Could you check a few things on this drawing? It's one solid part, dimensions in mm from its lowest x, y, z. Give positions to 0.01 mm unless a question says otherwise; leave off trailing zeros. Order: outer loops, then holes, each group sorted by start corner. A loop starts at its lowest first (then second) coordinate and runs counter-clockwise, first axis right, second up. Notation, with made-up numbers: (-33.5, -17) -> (-0.5, -17) arc R18 ccw to (-0.5, 10) -> close; hole circle Ø7 at (-7.75, 12.25). An arc over 180 degrees is marked (long way). Write each question's results on one line, items separated by ' | '.
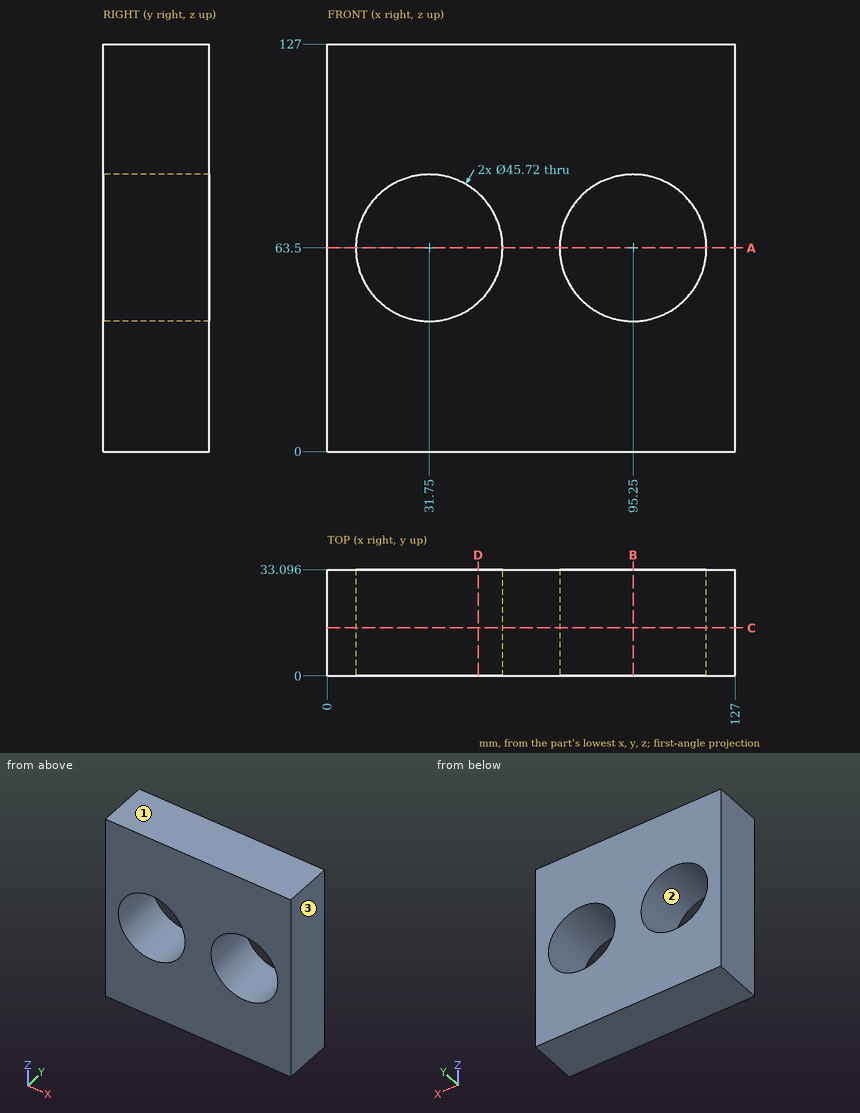
Q1. Thinking about a two-plate mould opening in Z: for the marked faces 1, 2 and 3, which applies, +Z half, -Z half, draft (parallel to the pull), parting line (faces both ways), or undercut?
Here are the results:
face 1: +Z half | face 2: undercut | face 3: draft
Q2. I'm going to push a flat-ended pin straight in: pin 1 Ø12 at (y, z) = (22, 77.5) entering from -X. Where does the tip first touch, or does it pass through?
Here are the results:
pin 1: stops at x = 0
Q3. Suppose I cut it at D-D on x = 47. Please give me the cut outline in (y, z), and give its area (3 significant figures).
Here are the results:
outline: (0, 0) -> (33.1, 0) -> (33.1, 46.47) -> (0, 46.47) -> close; (0, 80.53) -> (33.1, 80.53) -> (33.1, 127) -> (0, 127) -> close | area: 3,080 mm²
Q4. Suppose I cut it at B-B on x = 95.25. Please give me the cut outline in (y, z).
Here are the results:
outline: (0, 0) -> (33.1, 0) -> (33.1, 40.64) -> (0, 40.64) -> close; (0, 86.36) -> (33.1, 86.36) -> (33.1, 127) -> (0, 127) -> close
Q5. Suppose I cut it at A-A on z = 63.5. Please give me the cut outline in (x, y), and give its area (3 significant figures).
Here are the results:
outline: (0, 0) -> (8.89, 0) -> (8.89, 33.1) -> (0, 33.1) -> close; (54.61, 0) -> (72.39, 0) -> (72.39, 33.1) -> (54.61, 33.1) -> close; (118.11, 0) -> (127, 0) -> (127, 33.1) -> (118.11, 33.1) -> close | area: 1,180 mm²
Q6. I need wall thicknesses on line 1 along X through (y, z) = (10, 63); line 2 along X through (y, z) = (10.5, 44); line 3 along Z through (x, y) = (99.5, 31). Which ranges of each line are inside material? Lowest first, please.
Here are the results:
line 1: x = 0 to 8.9, 54.6 to 72.4, 118.1 to 127 | line 2: x = 0 to 19.82, 43.68 to 83.32, 107.18 to 127 | line 3: z = 0 to 41.04, 85.96 to 127
Q7. Suppose I cut it at C-C on y = 15. Please give me the cut outline in (x, z), and give its area (3 significant figures).
Here are the results:
outline: (0, 0) -> (127, 0) -> (127, 127) -> (0, 127) -> close; hole circle Ø45.72 at (31.75, 63.5); hole circle Ø45.72 at (95.25, 63.5) | area: 12,800 mm²
